from build123d import *

# Parameters (mm, degrees)
EXTRUDE_1_DEPTH     = 20
SKETCH_2_R          = 1.6
CUT_EXTRUDE_1_DEPTH = 60.634302209
FILLET_1_R          = 3.5
FILLET_2_R          = 0.5


with BuildPart() as part:
    # 草图1 → 凸台-拉伸1 (new body)
    with BuildSketch(Plane.XY):
        with BuildLine():
            Line((0, 0), (20, 0))
            Line((20, 0), (20, 30))
            Line((20, 30), (20, 52.5))
            Line((20, 52.5), (14.118252056, 52.5))
            ThreePointArc((14.118252056, 52.5), (10, 41.9), (5.881747944, 52.5))
            Line((5.881747944, 52.5), (0, 52.5))
            Line((0, 52.5), (0, 30))
            Line((0, 30), (0, 0))
        make_face()
    extrude(amount=EXTRUDE_1_DEPTH)

    # 草图2 → 切除-拉伸1 (cut, through all)
    with BuildSketch(Plane(origin=(20, 0, 0), x_dir=(0, 0, -1), z_dir=(1, 0, 0))):
        with Locations((-15, 24)):
            Circle(SKETCH_2_R)
        with Locations(Location((-15, 6, 0), (0, 0, 180))):
            Circle(SKETCH_2_R)
        with Locations((-5, 6)):
            Circle(SKETCH_2_R)
        with Locations(Location((-5, 24, 0), (0, 0, 180))):
            Circle(SKETCH_2_R)
    extrude(amount=-CUT_EXTRUDE_1_DEPTH, mode=Mode.SUBTRACT)

    # 圆角1
    fillet_1_edges = [part.edges().sort_by_distance(p)[0] for p in [
        (0, 52.5, 10),
        (20, 52.5, 10),
    ]]
    fillet(fillet_1_edges, radius=FILLET_1_R)

    # 圆角2
    fillet_2_edges = [part.edges().sort_by_distance(p)[0] for p in [
        (5.881747944, 52.5, 10),
        (14.118252056, 52.5, 10),
    ]]
    fillet(fillet_2_edges, radius=FILLET_2_R)


solid = part.part
Part model, mm, in its own coordinate system. Coordinates: 2 decimals unless noted, no trailing zeros. Order: outer loops, then holes, each group sorted by start corner. A loop starts at its lowest first (then second) coordinate and runs counter-clockwise, first axis right, second up. Notation, with made-up numbers: M 70.25,-17.5 L 124.25,-17.5 A16 ccw 124.25,-13.5 Z; hole C 59,67 d1. An arc over 180 degrees is marked long. Use a Markdown table: item, result.
(1) Cut at A-A on y = 48. Write the cut outline in (x, z), then the cut area to 3 significant figures.
A:
| item | result |
|---|---|
| outline | M 0,0 L 3.9,0 L 3.9,20 L 0,20 Z; M 16.1,0 L 20,0 L 20,20 L 16.1,20 Z |
| area | 156 mm^2 |
(2) Cut at B-B on x = 10. Write the cut outline in (y, z), then the cut area to 3 significant figures.
A:
| item | result |
|---|---|
| outline | M 0,0 L 41.9,0 L 41.9,20 L 0,20 Z; hole C 6,5 d3.2; hole C 6,15 d3.2; hole C 24,5 d3.2; hole C 24,15 d3.2 |
| area | 806 mm^2 |
(3) Flat gauge pins, fed straight in: pin 1 (1.9 mm diameter, centred on y = 6, z = 15, fed in from +X); pin 2 (2 mm diameter, centred on x = 11.5, z = 3, fed in from +Y). Where does each tip first touch, or does it go through?
A:
| item | result |
|---|---|
| pin 1 | passes through |
| pin 2 | stops at y = 42.44 |
(4) Cut at C-C on y = 6. Write the cut outline in (x, z).
A:
| item | result |
|---|---|
| outline | M 0,0 L 20,0 L 20,3.4 L 0,3.4 Z; M 0,6.6 L 20,6.6 L 20,13.4 L 0,13.4 Z; M 0,16.6 L 20,16.6 L 20,20 L 0,20 Z |
(5) Cut at D-D on z = 15. Write the cut outline in (x, y), then the cut area to 3 significant figures.
A:
| item | result |
|---|---|
| outline | M 0,0 L 20,0 L 20,4.4 L 0,4.4 Z; M 0,7.6 L 20,7.6 L 20,22.4 L 0,22.4 Z; M 0,25.6 L 20,25.6 L 20,49 A3.5 ccw 16.5,52.5 L 15.25,52.5 A0.5 ccw 14.85,51.7 A6.1 cw long 5.15,51.7 A0.5 ccw 4.75,52.5 L 3.5,52.5 A3.5 ccw 0,49 Z |
| area | 808 mm^2 |
(6) Probe L1, parallel to Y at x = 9, z = 5.25; L2, parallel to X at y = 48, z = 1.5; L3, parallel to Z at x = 9.75, y = 5.5. List the from-to ranges inside material, lowest first.
A:
| item | result |
|---|---|
| L1 | y = 0 to 4.42, 7.58 to 22.42, 25.58 to 41.98 |
| L2 | x = 0 to 3.9, 16.1 to 20 |
| L3 | z = 0 to 3.48, 6.52 to 13.48, 16.52 to 20 |
(7) Pull direction Z, two halves, no side cores. Call faces 1 (the cylindrical face through (10.14, 24.07, 16.6)), 2 (the cylindrical face through (10.19, 41.903, 9.86)), 3 (the flat face through (10, 27, 0)): released by +Z, released by -Z, zero draft, split by the parting line, or undercut.
A:
| item | result |
|---|---|
| face 1 | undercut |
| face 2 | zero draft |
| face 3 | released by -Z |
